Here's how the part is built. I have some questions about the finished solid (model axes, mm). Round coordinates to 2 decimals unless told otherwise and drop trailing zeros. Loops run counter-clockwise (first coordinate to the right, second up) from the corner with the lowest first, then second, coordinate; pieces in that order, holes last. Notation, with made-up numbers: (-2, 6.5) - (44, 6.5) arc R10 cw to (44, 11.5) - close; hole circle Ø11 at (4, -16). An arc over 180 degrees is marked (long way). Answer as a JSON object with one key per item and string values. Group by question number.
1) I want a section at C-C, the plane x = -112.5. Please give me the cut outline in (y, z) (1 decimal).
2) If I drill on line 1 along X through (y, z) = (47, -3); line 2 along X through (y, z) = (44.5, -0.9); line 3 along X through (y, z) = (62, -0.75), over which ranges is the centre line in solid material (lowest first)? Write a range as [from, to].
3) Will these pins go through, and if not, where does the flat tip stop? P1, Ø16.5, axis at x = -31.75, y = 60.325, coming from the +Z side; P2, Ø3, axis at x = -103.251, y = 22.225, coming from the -Z side.
4) I want a section at A-A, the plane y = 45.72. Please give me the cut outline in (x, z) (3 decimals), then the cut area to 3 significant figures.
5) I want a section at D-D, the plane z = -1.1. Give the number of separate pieces and of enclosed holes in the cut face, then the cut area to 3 significant figures.
6) If we mould it in two halves opening along Y, with no side actions, what happens to faces 1 (the face through (-113.396, 26.947, -1.565)), 2 (the face through (-74, 76.2, -2)), 3 (the face through (0, 38, -2)), 4 (the face through (-74, 0, -2))? For each: pulls with the +Y half, pulls with the -Y half, needs draft (parallel to the pull), parting line crosses it, or undercut.
7) I want a section at B-B, the plane x = -72.39. Please give me the cut outline in (y, z) (3 decimals), then the cut area to 3 significant figures.
from build123d import *

# Parameters (mm, degrees)
SKETCH1_W                    = 146.05
SKETCH1_H                    = 76.2
BOSS_EXTRUDE1_DEPTH          = 3.175
F_6_CLEARANCE_HOLE1_D        = 4.3053
F_1_2_0_5_DIAMETER_HOLE1_D   = 12.7
F_3_8_0_375_DIAMETER_HOLE1_D = 9.525
F_1_8_0_125_DIAMETER_HOLE1_D = 3.175


with BuildPart() as part:
    # Sketch1 → Boss-Extrude1 (new body)
    with BuildSketch(Plane.XY):
        with Locations((-73.025, 38.1)):
            Rectangle(SKETCH1_W, SKETCH1_H)
    extrude(amount=-BOSS_EXTRUDE1_DEPTH)

    # #6 Clearance Hole1 (through all)
    with Locations(Plane(origin=(0, 0, -3.175), x_dir=(-1, 0, 0), z_dir=(0, 0, -1))):
        with Locations((4.8895, 61.9125), (4.8895, 14.2875), (141.1605, 14.2875), (141.1605, 61.9125), (128.016, 45.72), (18.034, 45.72)):
            Hole(F_6_CLEARANCE_HOLE1_D / 2)

    # 1/2 (0.5) Diameter Hole1 (through all)
    with Locations(Plane(origin=(0, 0, -3.175), x_dir=(-1, 0, 0), z_dir=(0, 0, -1))):
        with Locations((31.75, 60.325), (72.39, 57.658), (112.776, 60.325)):
            Hole(F_1_2_0_5_DIAMETER_HOLE1_D / 2)

    # 3/8 (0.375) Diameter Hole1 (through all)
    with Locations(Plane(origin=(0, 0, -3.175), x_dir=(-1, 0, 0), z_dir=(0, 0, -1))):
        with Locations((38.1, 22.225), (112.776, 22.225)):
            Hole(F_3_8_0_375_DIAMETER_HOLE1_D / 2)

    # 1/8 (0.125) Diameter Hole1 (through all)
    with Locations(Plane(origin=(0, 0, -3.175), x_dir=(-1, 0, 0), z_dir=(0, 0, -1))):
        with Locations((31.75, 69.699492067), (112.695431447, 69.699492067), (103.251, 22.225), (31.98067476, 16.130346764)):
            Hole(F_1_8_0_125_DIAMETER_HOLE1_D / 2)


solid = part.part
Outcome:
{
 "1": {"outline": "(0, -3.2) - (17.5, -3.2) - (17.5, 0) - (0, 0) - close; (27, -3.2) - (54, -3.2) - (54, 0) - (27, 0) - close; (66.7, -3.2) - (68.1, -3.2) - (68.1, 0) - (66.7, 0) - close; (71.3, -3.2) - (76.2, -3.2) - (76.2, 0) - (71.3, 0) - close"},
 "2": {"line 1": "[-146.05, -129.75], [-126.29, -19.76], [-16.3, 0]", "line 2": "[-146.05, -129.79], [-126.24, -19.81], [-16.26, 0]", "line 3": "[-146.05, -143.31], [-139.01, -118.9], [-106.65, -77.02], [-67.76, -37.88], [-25.62, -7.04], [-2.74, 0]"},
 "3": {"P1": "z = 0", "P2": "through"},
 "4": {"outline": "(-146.05, -3.175) - (-130.169, -3.175) - (-130.169, 0) - (-146.05, 0) - close; (-125.863, -3.175) - (-20.187, -3.175) - (-20.187, 0) - (-125.863, 0) - close; (-15.881, -3.175) - (0, -3.175) - (0, 0) - (-15.881, 0) - close", "area": "436 mm^2"},
 "5": {"separate pieces": "1", "enclosed holes": "15", "area": "10,500 mm^2"},
 "6": {"face 1": "undercut", "face 2": "pulls with the +Y half", "face 3": "needs draft", "face 4": "pulls with the -Y half"},
 "7": {"outline": "(0, -3.175) - (51.308, -3.175) - (51.308, 0) - (0, 0) - close; (64.008, -3.175) - (76.2, -3.175) - (76.2, 0) - (64.008, 0) - close", "area": "202 mm^2"}
}
